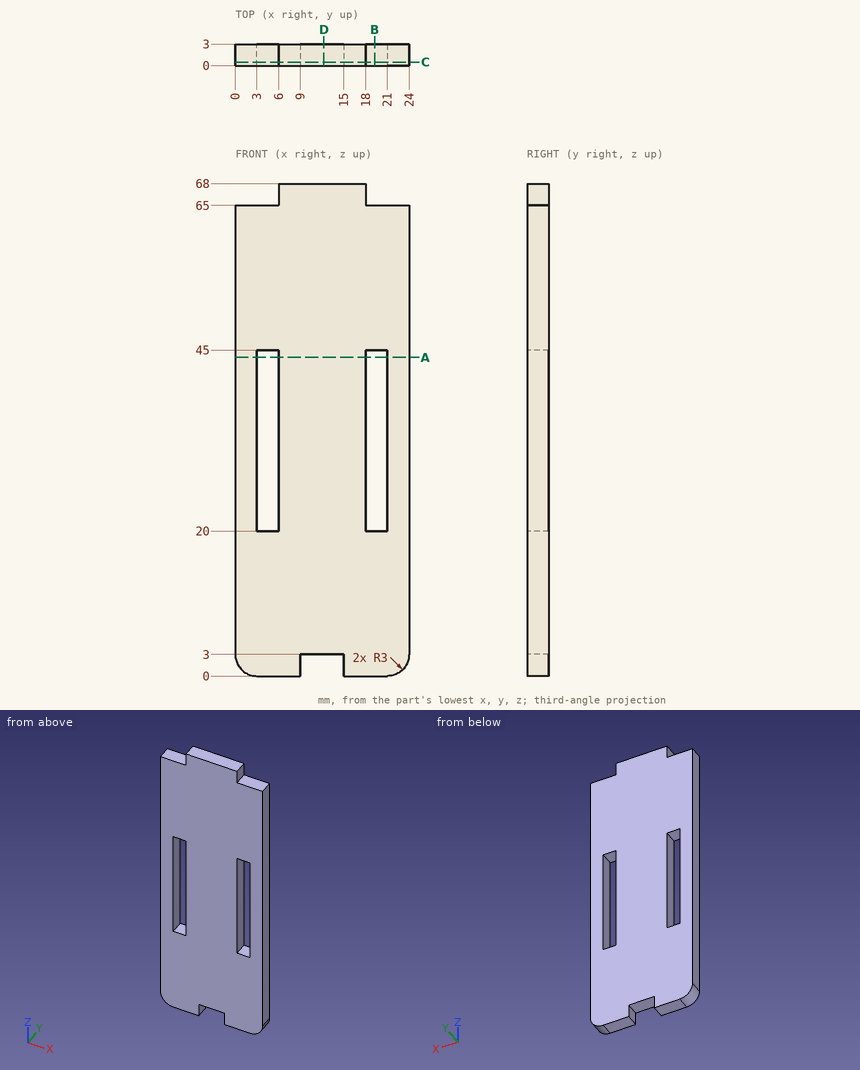
Part print with two shaded views. Sizes in mm from the minimum x, y, z corner. Round coordinates to 2 decimals unless told otherwise and drop trailing zeros. Loops run counter-clockwise (first coordinate to the right, second up) from the corner with the lowest first, then second, coordinate; pieces in that order, holes last. Notation, with made-up numbers: M -30.75,41.5 L -26.75,41.5 A15 cw -26.75,70.5 Z; hole C -8,72.25 d7. An arc over 180 degrees is marked long. Put each result on its own line as item: value. Start each with the question number.
Item 1: Cut at B-B (x = 19.25). List the corners of the cut face in (y, z).
Item 2: Drop flat-ended pins along their axis: P1, Ø0.9, axis at x = 19, y = 1, coming from the +Z side; P2, Ø1.5, axis at x = 13.5, y = 1, coming from the -Z side; P3, Ø1.5, axis at y = 2, z = 1, coming from the -X side. Give the stop position or say it passes through.
Item 3: Drill centre lines: line 1 along X through (y, z) = (1, 39); line 2 along Z through (x, y) = (19.5, 1.85); line 3 along Z through (x, y) = (10, 2.8). Where is each one in solid material? Low to high.
Item 4: Cut at C-C (y = 0.5). List the corners of the cut face in (x, z).
Item 5: Cut at D-D (x = 12.25). List the corners of the cut face in (y, z), then the cut area to 3 significant figures.
Item 6: Cut at A-A (z = 44). List the corners of the cut face in (x, y).
Answer block:
1. outline: M 0,0 L 3,0 L 3,20 L 0,20 Z; M 0,45 L 3,45 L 3,65 L 0,65 Z
2. P1: z = 65
2. P2: z = 3
2. P3: x = 0.27
3. line 1: 0 to 3, 6 to 18, 21 to 24
3. line 2: 0 to 20, 45 to 65
3. line 3: 3 to 68
4. outline: M 0,3 A3 ccw 3,0 L 9,0 L 9,3 L 15,3 L 15,0 L 21,0 A3 ccw 24,3 L 24,65 L 18,65 L 18,68 L 6,68 L 6,65 L 0,65 Z; hole M 3,20 L 6,20 L 6,45 L 3,45 Z; hole M 18,20 L 21,20 L 21,45 L 18,45 Z
5. outline: M 0,3 L 3,3 L 3,68 L 0,68 Z
5. area: 195 mm2
6. outline: M 0,0 L 3,0 L 3,3 L 0,3 Z; M 6,0 L 18,0 L 18,3 L 6,3 Z; M 21,0 L 24,0 L 24,3 L 21,3 Z
